Print and shaded views of the part. All mm, measured from the part's lowest x, y and z. Round coordinates to 2 decimals unless told otherwise and drop trailing zeros. Write each loop counter-clockwise with the first axis right and the second up, starting at its lowest first coordinate (ties: lowest second). Pieces come first, ordered by that corner, then holes. Notation, with made-up numbers: (55, 59) -> (70, 59) arc R15 ccw to (70, 65) -> close; hole circle Ø8 at (80, 69). An arc over 180 degrees is marked (long way). Return JSON: item names as keys, results as strings. Group by question number.
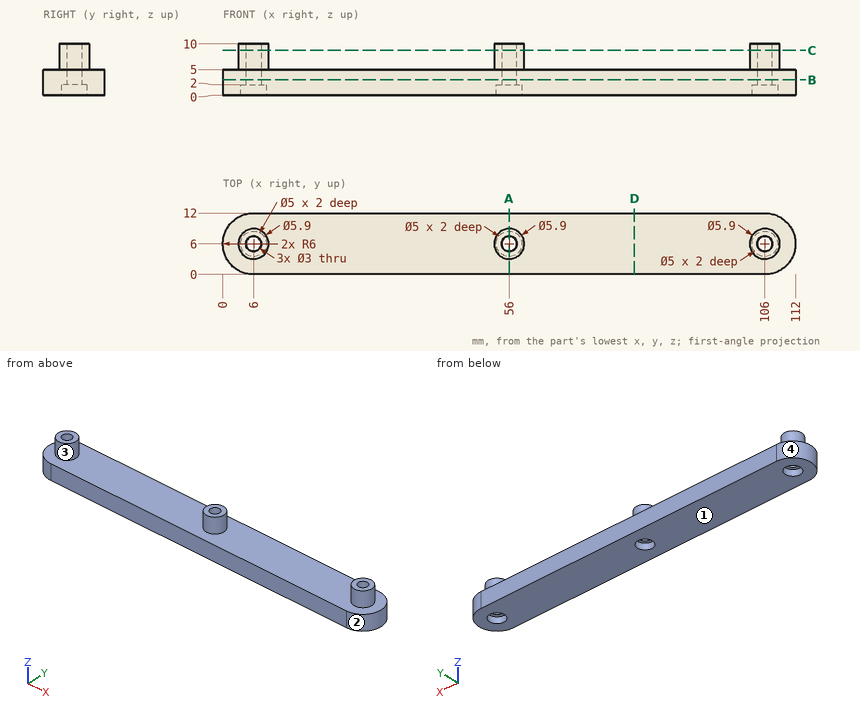
Item 1: Flat gauge pins, fed straight in: P1, Ø2.5, axis at x = 106.5, y = 5.5, coming from the -Z side; P2, Ø6.5, axis at x = 106, y = 6, coming from the +Z side; P3, Ø5, axis at x = 87, z = 8.5, coming from the +Y side; P4, Ø4, axis at y = 2.5, z = 7.5, coming from the -X side. Where does each tip first touch, or does it go through?
Item 2: Cut at C-C (z = 8.75). Write the cut outline in (x, y), then the cut area to 3 significant figures.
Item 3: Cut at D-D (x = 80.5). Write the cut outline in (y, z), then the cut area to 3 significant figures.
Item 4: Two-plate mould, pull along X, no slides. Class the marked faces 1, 2, 3 and 4: released by +X, released by -X, zero draft, split by the parting line, or undercut.
Item 5: Cut at A-A (x = 56). Write the cut outline in (y, z), then the cut area to 3 significant figures.
Item 6: Wall check: L1, parallel to X at y = 6, z = 4.75; L2, parallel to Y at x = 56, z = 1.15; L3, parallel to Y at x = 56, z = 5.75. Give the ranges that are in metal, low to high.
Item 7: Cut at B-B (z = 3). Write the cut outline in (x, y).
Checks:
{
 "1": {"P1": "stops at z = 2", "P2": "stops at z = 10", "P3": "passes through", "P4": "stops at x = 3.46"},
 "2": {"outline": "circle Ø5.9 at (6, 6); circle Ø5.9 at (56, 6); circle Ø5.9 at (106, 6); hole circle Ø3 at (6, 6); hole circle Ø3 at (56, 6); hole circle Ø3 at (106, 6)", "area": "60.8 mm2"},
 "3": {"outline": "(0, 0) -> (12, 0) -> (12, 5) -> (0, 5) -> close", "area": "60.0 mm2"},
 "4": {"face 1": "zero draft", "face 2": "released by +X", "face 3": "undercut", "face 4": "released by -X"},
 "5": {"outline": "(0, 0) -> (3.5, 0) -> (3.5, 2) -> (4.5, 2) -> (4.5, 10) -> (3.05, 10) -> (3.05, 5) -> (0, 5) -> close; (7.5, 2) -> (8.5, 2) -> (8.5, 0) -> (12, 0) -> (12, 5) -> (8.95, 5) -> (8.95, 10) -> (7.5, 10) -> close", "area": "55.5 mm2"},
 "6": {"L1": "x = 0 to 4.5, 7.5 to 54.5, 57.5 to 104.5, 107.5 to 112", "L2": "y = 0 to 3.5, 8.5 to 12", "L3": "y = 3.05 to 4.5, 7.5 to 8.95"},
 "7": {"outline": "(6, 0) -> (106, 0) arc R6 ccw to (106, 12) -> (6, 12) arc R6 ccw to start; hole circle Ø3 at (6, 6); hole circle Ø3 at (56, 6); hole circle Ø3 at (106, 6)"}
}
